from build123d import *

# Parameters (mm, degrees)
ESBO_O2_R                = 2
RESSALTO_EXTRUS_O1_DEPTH = 1.2
FILETE1_R                = 1
FILETE2_R                = 1
ESCALA1_SCALE            = 0.571428571


with BuildPart() as part:
    # Esboço1 → Revolução1 (revolve)
    with BuildSketch(Plane.XY):
        with BuildLine():
            Line((0, 0), (-16.1, 0))
            Line((-16.1, 0), (-16.1, -1.2))
            Line((-16.1, -1.2), (-14.25, -1.2))
            Line((-14.25, -1.2), (-14.25, -9.358571571))
            ThreePointArc((-14.25, -9.358571571), (-13.469544457, -13.231554918), (-11.25, -16.5))
            ThreePointArc((-11.25, -16.5), (-9.286251005, -16.915617464), (-7.5, -16))
            ThreePointArc((-7.5, -16), (-4.506939094, -19.635408641), (0, -21))
            Line((0, -21), (0, 0))
        make_face()
    revolve(axis=Axis((0, 0, 0), (0, 1, 0)))

    # Esboço2 → Ressalto-extrusão1 (add)
    with BuildSketch(Plane(origin=(0, 0, 0), x_dir=(1, 0, 0), z_dir=(0, 1, 0))):
        with BuildLine():
            Line((13.032253871, 9.453589744), (3.763973944, 22.230384615))
            ThreePointArc((3.763973944, 22.230384615), (0, 24.15), (-3.763973944, 22.230384615))
            Line((-3.763973944, 22.230384615), (-13.032253871, 9.453589744))
            ThreePointArc((-13.032253871, 9.453589744), (0, 16.1), (13.032253871, 9.453589744))
        make_face()
        with Locations((0, 19.5)):
            Circle(ESBO_O2_R, mode=Mode.SUBTRACT)
        with BuildLine():
            Line((3.763973944, -22.230384615), (13.032253871, -9.453589744))
            ThreePointArc((13.032253871, -9.453589744), (0, -16.1), (-13.032253871, -9.453589744))
            Line((-13.032253871, -9.453589744), (-3.763973944, -22.230384615))
            ThreePointArc((-3.763973944, -22.230384615), (0, -24.15), (3.763973944, -22.230384615))
        make_face()
        with Locations((0, -19.5)):
            Circle(ESBO_O2_R, mode=Mode.SUBTRACT)
    extrude(amount=-RESSALTO_EXTRUS_O1_DEPTH)

    # Esboço3 → Corte-Revolução1 (revolve, cut)
    with BuildSketch(Plane(origin=(0, 0, 0), x_dir=(0, 0, -1), z_dir=(1, 0, 0))):
        with BuildLine():
            Line((-12.5, 0), (-12.5, -9))
            ThreePointArc((-12.5, -9), (-6.786587677, -4.882109006), (0, -3))
            Line((0, -3), (0, 0))
            Line((0, 0), (-12.5, 0))
        make_face()
    revolve(axis=Axis((0, 0, 0), (0, -1, 0)), mode=Mode.SUBTRACT)

    # Filete1
    filete1_edges = [part.edges().sort_by_distance(p)[0] for p in [
        (0, 0, -12.5),
    ]]
    fillet(filete1_edges, radius=FILETE1_R)

    # Filete2
    filete2_edges = [part.edges().sort_by_distance(p)[0] for p in [
        (14.25, -1.2, 0),
    ]]
    fillet(filete2_edges, radius=FILETE2_R)


with BuildPart() as part_1:
    # Escala1: scaled about (0, -9.829669645, 0)
    add(part.part.scale(ESCALA1_SCALE).moved(Location((0, -4.212715562, 0))))


solid = part_1.part
The listing builds one solid part. Answer for the finished solid, in the listing's coordinates (mm). A direction names the side the tool comes from. Coordinates: 2 decimals unless noted, no trailing zeros. Order: outer loops, then holes, each group sorted by start corner. A loop starts at its lowest first (then second) coordinate and runs counter-clockwise, first axis right, second up.
Q1. Which of the six approach directions +Z, -Z, +X, -X, +Y, -Y give full straight-line access (tool end or side, diameter ignored) to faces 4 (the face through (-7.767, -7.544, 2.446)), 5 (the face through (-0.25, -4.55, 12.26))?
Q2. A cutting plane is placed at B-B, the plane y = -6.5. State how many separate pieces and enclosed holes the cut face has, and give its area (3 significant figures).
Q3. For a pull along X with two mould halves and no side action, classify faces 1 (the face through (-9, -4.898, 0)), 2 (the face through (-9.2, -4.6, -0.1)), 3 (the face through (-7.082, -7.102, -0.93)) as pulls with the +X half, pulls with the -X half, needs draft (parallel to the pull), parting line crosses it, or undercut.
Q4. Given P1, Ø4, axis at x = 1.5, y = -9.5, coming from the -Z side; P2, Ø1, axis at x = -6, y = -13, coming from the -Z side; P3, Ø1.4, axis at x = 0, z = 11.14, coming from the -Y side; P4, Ø4, axis at x = -0.5, z = -8, coming from the -Y side, each flat-ended and moving along its own axis, determine where each tip first touches the part or whether it passes through.
Q5. A cutting plane is placed at A-A, the plane z = -11.5. Write down the section's boundary in (x, y), and give its area (3 significant figures).
Q6. Consider line 1 (Z direction, x = 0, y = -4.65); line 2 (Z direction, x = 0, y = -4.35); line 3 (Z direction, x = -1.5, y = -7.5). Determine where each line is inside the solid, lowest interval first.
Q7. A cutting plane is placed at C-C, the plane y = -15.25. Write down the section's boundary in (x, z), and give its area (3 significant figures).
Answers follow:
1. face 4: -Y
1. face 5: +Y, -Y
2. separate pieces: 2
2. enclosed holes: 1
2. area: 70.2 mm2
3. face 1: needs draft
3. face 2: pulls with the -X half
3. face 3: undercut
4. P1: stops at z = -8.14
4. P2: stops at z = -4.53
4. P3: passes through
4. P4: stops at y = -13.82
5. outline: (-3.02, -4.9) - (-1.09, -4.9) - (-1.09, -4.21) - (-3.02, -4.21) - close; (1.09, -4.9) - (3.02, -4.9) - (3.02, -4.21) - (1.09, -4.21) - close
5. area: 2.66 mm2
6. line 1: z = -13.8 to -12.29, -10 to -7.16, 7.16 to 10, 12.29 to 13.8
6. line 2: z = -13.8 to -12.29, -10 to -7.34, 7.34 to 10, 12.29 to 13.8
6. line 3: z = -8 to -6.98, -4.56 to 4.56, 6.98 to 8
7. outline: circle Ø5.66 at (0, 0)
7. area: 25.2 mm2
